CAD build for the part. Positions are in the model's coordinates, mm. Face numbers are marked on the shaded views. A direction names the side the tool comes from. Round coordinates to 2 decimals unless told otherwise and drop trailing zeros. Loops run counter-clockwise (first coordinate to the right, second up) from the corner with the lowest first, then second, coordinate; pieces in that order, holes last. Notation, with made-up numbers: M 29.5,44.25 L 60.5,44.25 A27 ccw 60.5,80.25 Z; hole C -32,14.5 d11. An arc over 180 degrees is marked long. Use one line per item in the form item = value.
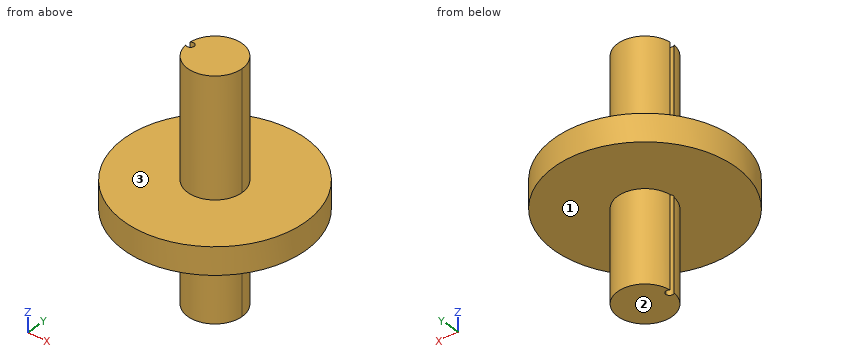
from build123d import *

# Parameters (mm, degrees)
F0_R     = 10
F1_DEPTH = 3
F0_R_2   = 1.65
F2_DEPTH = 16
F3_DEPTH = 10


with BuildPart() as f1:
    # F0 (on Top) → F1 (new body)
    with BuildSketch(Plane.XY):
        Circle(F0_R)
        with BuildLine():
            ThreePointArc((-2.987037, 0.278585), (0.139443, 2.996758), (3, 0))
            ThreePointArc((3, 0), (0.139443, -2.996758), (-2.987037, -0.278585))
            ThreePointArc((-2.987037, -0.278585), (-3.1, 0), (-2.987037, 0.278585))
        make_face(mode=Mode.SUBTRACT)
    extrude(amount=F1_DEPTH)

    # F0 (on Top) → F2 (join)
    with BuildSketch(Plane.XY):
        with BuildLine():
            ThreePointArc((-2.987037, -0.278585), (0.139443, -2.996758), (3, 0))
            ThreePointArc((3, 0), (0.139443, 2.996758), (-2.987037, 0.278585))
            ThreePointArc((-2.987037, 0.278585), (-2.549692, 0.370685), (-2.3, 0))
            ThreePointArc((-2.3, 0), (-2.549692, -0.370685), (-2.987037, -0.278585))
        make_face()
        Circle(F0_R_2, mode=Mode.SUBTRACT)
        Circle(F0_R_2)
    extrude(amount=F2_DEPTH)

    # F0 (on Top) → F3 (join)
    with BuildSketch(Plane.XY):
        with BuildLine():
            ThreePointArc((-2.987037, -0.278585), (0.139443, -2.996758), (3, 0))
            ThreePointArc((3, 0), (0.139443, 2.996758), (-2.987037, 0.278585))
            ThreePointArc((-2.987037, 0.278585), (-2.549692, 0.370685), (-2.3, 0))
            ThreePointArc((-2.3, 0), (-2.549692, -0.370685), (-2.987037, -0.278585))
        make_face()
        Circle(F0_R_2, mode=Mode.SUBTRACT)
        Circle(F0_R_2)
    extrude(amount=-F3_DEPTH)


solid = f1.part
1. Tool access for the marked faces 1, 2 and 3: list every direction of +Z, -Z, +X, -X, +Y, -Y with a clear straight run to the whole face (end or side of a thin tool).
Completed:
face_1 = -Z
face_2 = -Z, +X, -X, +Y, -Y
face_3 = +Z
2. Drop flat-ended pins along their axis: P1, Ø6, axis at x = -2, z = -4.5, coming from the +Y side; P2, Ø6, axis at x = 4.5, z = 9, coming from the +Y side; P3, Ø1, axis at x = -7.5, y = -2, coming from the -Z side. Give the stop position or say it passes through.
Completed:
P1 = 3
P2 = 2.6
P3 = 0
3. Cut at C-C on z = 0.75. Write the cut outline in (x, y), and give its area (3 significant figures).
Completed:
outline = C 0,0 d20; hole C -2.7,0 d0.8
area = 314 mm2
4. Cut at A-A on x = 0. Write the cut outline in (y, z), and give its area (3 significant figures).
Completed:
outline = M -10,0 L -3,0 L -3,-10 L 3,-10 L 3,0 L 10,0 L 10,3 L 3,3 L 3,16 L -3,16 L -3,3 L -10,3 Z
area = 198 mm2
5. Cut at B-B on y = -1.25. Write the cut outline in (x, z), and give its area (3 significant figures).
Completed:
outline = M -9.92,0 L -2.73,0 L -2.73,-10 L 2.73,-10 L 2.73,0 L 9.92,0 L 9.92,3 L 2.73,3 L 2.73,16 L -2.73,16 L -2.73,3 L -9.92,3 Z
area = 185 mm2
6. Probe line 1 along Z through (x, y) = (-3.75, -3.75); line 2 along X through (y, z) = (-1.25, -4.5); line 3 along X through (y, z) = (2.75, 7.5). List the from-to ranges inside material, lowest first. Write a range as from..to.
Completed:
line_1 = 0..3
line_2 = -2.73..2.73
line_3 = -1.2..1.2
